```python
from build123d import *

# Parameters (mm, degrees)
F1_DEPTH = 25
F2_R     = 1.6
F3_DEPTH = 32


with BuildPart() as f1:
    # F0 (on Right) → F1 (new body)
    with BuildSketch(Plane.YZ):
        with BuildLine():
            ThreePointArc((4.861622, 17.075245), (0.592168, 1.441825), (-3.681383, 17.074125))
            Line((-3.681383, 17.074125), (-13.558886, 17.074125))
            Line((-13.558886, 17.074125), (-13.558383, -8.158872))
            Line((-13.558383, -8.158872), (14.738216, -8.158172))
            Line((14.738216, -8.158172), (14.739622, 17.075245))
            Line((14.739622, 17.075245), (4.861622, 17.075245))
        make_face()
    extrude(amount=F1_DEPTH)

    # F2 (on face) → F3 (cut)
    with BuildSketch(Plane(origin=(0, -13.558546, -0.00027), x_dir=(1, 0, 0), z_dir=(0, -1, -2e-05))):
        with Locations((12.5, -5.28356)):
            Circle(F2_R)
    extrude(amount=-F3_DEPTH, mode=Mode.SUBTRACT)


solid = f1.part
```
CAD build for the part. Positions are in the model's coordinates, mm. Give positions to 0.01 mm unless a question says otherwise; leave off trailing zeros. Write each loop counter-clockwise with the first axis right and the second up, starting at its lowest first coordinate (ties: lowest second). Pieces come first, ordered by that corner, then holes. Notation, with made-up numbers: M -39,-34 L -26,-34 A7 cw -26,-24 Z; hole C 49,-35.5 d11. An arc over 180 degrees is marked long. Return JSON: item names as keys, results as strings. Group by question number.
(1) Flat gauge pin, fed straight in: pin 1 Ø13.5 at (y, z) = (0.59, 9.84) entering from +X. Where does the tip first touch, or does it go through?
(2) Band-saw the part on B-B (z = 4.75). Give the cut face in (x, y).
(3) Mould opens along X. For faces 1 (the face through (25, -3, 2)), 2 (the face through (10.9, 0.39, -5.21)), 3 (the face through (12, -9, 17.074)), 4 (the face through (0, -3, 2)) say: pulls with the +X half, pulls with the -X half, needs draft (parallel to the pull), parting line crosses it, or undercut.
(4) Band-saw the part on D-D (z = 12.25). Give the cut face in (x, y).
(5) Band-saw the part on C-C (y = 5.75). State how many separate pieces and enclosed holes the cut face has, and give its area (3 significant figures).
(6) Band-saw the part on A-A (x = 12.5). Give the cut face in (y, z).
(7) Drill centre lines: L1, parallel to Y at x = 22.5, z = 9.75; L2, parallel to Z at x = 12.5, y = -4.75; L3, parallel to Z at x = 12.5, y = -5.5. Where is each one in solid material? Low to high. Write a range as [from, to].
Entries:
{
 "1": {"pin 1": "passes through"},
 "2": {"outline": "M 0,-13.56 L 25,-13.56 L 25,-6.09 L 0,-6.09 Z; M 0,7.27 L 25,7.27 L 25,14.74 L 0,14.74 Z"},
 "3": {"face 1": "pulls with the +X half", "face 2": "undercut", "face 3": "needs draft", "face 4": "pulls with the -X half"},
 "4": {"outline": "M 0,-13.56 L 25,-13.56 L 25,-7.46 L 0,-7.46 Z; M 0,8.64 L 25,8.64 L 25,14.74 L 0,14.74 Z"},
 "5": {"separate pieces": "2", "enclosed holes": "1", "area": "291 mm^2"},
 "6": {"outline": "M -13.56,-8.16 L 14.74,-8.16 L 14.74,-6.88 L -13.56,-6.88 Z; M -13.56,-3.68 L 14.74,-3.68 L 14.74,17.08 L 4.86,17.08 A8.4 cw long -3.68,17.07 L -13.56,17.07 Z"},
 "7": {"L1": "y = [-13.56, -7.81], [8.99, 14.74]", "L2": "z = [-8.16, -6.88], [-3.68, 3.36], [16.33, 17.07]", "L3": "z = [-8.16, -6.88], [-3.68, 4.06], [15.63, 17.07]"}
}
